Answer from the drawing. Dimensions are ordinates in mm from the lowest x, y and z of the part. Round coordinates to 2 decimals unless told otherwise and drop trailing zeros. Loops run counter-clockwise (first coordinate to the right, second up) from the corner with the lowest first, then second, coordinate; pieces in that order, holes last. Notation, with made-up numbers: (-3.75, 66) -> (5.25, 66) arc R28 ccw to (5.25, 92) -> close; hole circle Ø10 at (80.25, 65). An arc over 180 degrees is marked (long way). Use CSV: the item, a comma, the result in double quotes. Start each with the question number.
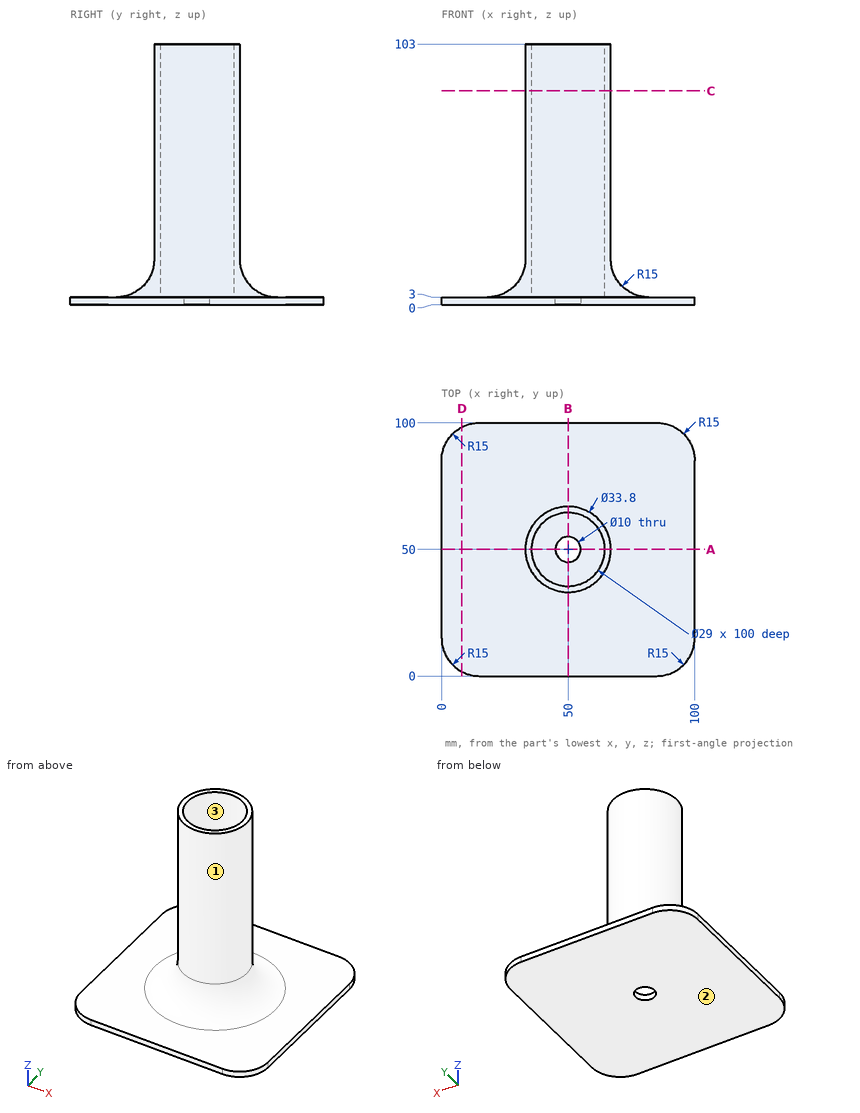
Q1. Section D-D, the plane x = 8 is taken. Write down the section's boundary in (y, z).
Q2. Straight lines are drawn through the part: line 1 (Y direction, x = 49.5, z = 26); line 2 (Z direction, x = 86, y = 30); line 3 (Y direction, x = 50, z = 1.85). For each, find the intervals that lie inside material, in ascending order. Write a range as from..to.
Q3. Section A-A, the plane y = 50 is taken. Write down the section's boundary in (x, z).
Q4. Section C-C, the plane z = 84.5 is taken. Write down the section's boundary in (x, y), and give its area (3 significant figures).
Q5. Each of these flat-tipped pins is pushed along its axis until it touches: pin 1 (6 mm diameter, centred on y = 44, z = 85.5, fed in from -X); pin 2 (14.5 mm diameter, centred on x = 52, y = 54, fed in from +Z); pin 3 (6 mm diameter, centred on x = 45, z = 82, fed in from +Y). Where does it stop, or does it pass through?
Q6. For a pull along X with two mould halves and no side action, classify the marked faces 1, 2 and 3 as pulls with the +X half, pulls with the -X half, needs draft (parallel to the pull), parting line crosses it, or undercut.
Report:
1,outline,"(1.73, 0) -> (98.27, 0) -> (98.27, 3) -> (1.73, 3) -> close"
2,line 1,"y = 33.11..35.51, 64.49..66.89"
2,line 2,"z = 0..3"
2,line 3,"y = 0..45, 55..100"
3,outline,"(0, 0) -> (45, 0) -> (45, 3) -> (35.5, 3) -> (35.5, 103) -> (33.1, 103) -> (33.1, 18) arc R15 cw to (18.1, 3) -> (0, 3) -> close; (55, 0) -> (100, 0) -> (100, 3) -> (81.9, 3) arc R15 cw to (66.9, 18) -> (66.9, 103) -> (64.5, 103) -> (64.5, 3) -> (55, 3) -> close"
4,outline,"circle Ø33.8 at (50, 50); hole circle Ø29 at (50, 50)"
4,area,"237 mm²"
5,pin 1,"stops at x = 33.37"
5,pin 2,"stops at z = 3"
5,pin 3,"stops at y = 66.78"
6,face 1,"parting line crosses it"
6,face 2,"needs draft"
6,face 3,"undercut"
